Source: CAD feature listing. Evaluate the final solid. Frame: model axes, mm. A direction names the side the tool comes from. Coordinates: 2 decimals unless noted, no trailing zeros. Write each loop counter-clockwise with the first axis right and the second up, starting at its lowest first coordinate (ties: lowest second). Pieces come first, ordered by that corner, then holes. Notation, with made-up numbers: (71.5, -29.75) - (114.5, -29.75) arc R19 ccw to (114.5, -1.75) - close; hole circle Ø11 at (64, 53). An arc over 180 degrees is marked (long way). One line per item, written item: value.
from build123d import *

# Parameters (mm, degrees)
F0_W      = 42
F0_H      = 42
F1_DEPTH  = 39
F2_R      = 16
F3_DEPTH  = 22.1
F4_R      = 10
F5_DEPTH  = 3
F6_R      = 3
F7_DEPTH  = 16.3
F8_SIZE   = 5
F10_DEPTH = 12
F12_DEPTH = 3
F14_D     = 2.5
F14_DEPTH = 7
F14_TIP   = 0.7510757738


with BuildPart() as f1:
    # F0 (on Front) → F1 (new body)
    with BuildSketch(Plane.XZ):
        Rectangle(F0_W, F0_H)
    extrude(amount=F1_DEPTH)

    # F2 (on face) → F3 (join)
    with BuildSketch(Plane.XZ.offset(39)):
        Circle(F2_R)
    extrude(amount=F3_DEPTH)

    # F4 (on face) → F5 (join)
    with BuildSketch(Plane.XZ.offset(61.1)):
        Circle(F4_R)
    extrude(amount=F5_DEPTH)

    # F6 (on face) → F7 (join)
    with BuildSketch(Plane.XZ.offset(64.1)):
        Circle(F6_R)
    extrude(amount=F7_DEPTH)

    # F8
    f8_edges = [f1.edges().sort_by_distance(p)[0] for p in [
        (-21, -19.5, 21),
        (21, -19.5, 21),
        (21, -19.5, -21),
        (-21, -19.5, -21),
    ]]
    chamfer(f8_edges, length=F8_SIZE)

    # F9 (on face) → F10 (cut)
    with BuildSketch(Plane.XZ.offset(80.4)):
        with BuildLine():
            Line((-1.6583123952, 2.5), (1.6583123952, 2.5))
            ThreePointArc((1.6583123952, 2.5), (0, 3), (-1.6583123952, 2.5))
        make_face()
    extrude(amount=-F10_DEPTH, mode=Mode.SUBTRACT)

    # F11 (on face) → F12 (cut, through all)
    with BuildSketch(Plane.XZ.offset(64.1)):
        with BuildLine():
            Line((3.2817540292, 9.4461680322), (9.4461680322, 3.2817540292))
            ThreePointArc((9.4461680322, 3.2817540292), (7.0710678119, 7.0710678119), (3.2817540292, 9.4461680322))
        make_face()
        with BuildLine():
            ThreePointArc((-9.4461680322, -3.2817540292), (-7.0710678119, -7.0710678119), (-3.2817540292, -9.4461680322))
            Line((-3.2817540292, -9.4461680322), (-9.4461680322, -3.2817540292))
        make_face()
    extrude(amount=-F12_DEPTH, mode=Mode.SUBTRACT)

    # F14
    with Locations(Plane.XZ.offset(61.1)):
        with Locations((0, 13), (-13, 0), (0, -13), (13, 0)):
            Hole(F14_D / 2, depth=F14_DEPTH)
            with Locations((0, 0, -(F14_DEPTH + F14_TIP / 2))):  # 118° drill point
                Cone(0, F14_D / 2, F14_TIP, mode=Mode.SUBTRACT)


solid = f1.part
1) Section query A-A on y = -63. Output: boundary loops of the cut face in (x, z), then the cut area to 3 significant figures.
Values found:
outline: (-9.45, -3.28) - (-3.28, -9.45) arc R10 ccw to (9.45, 3.28) - (3.28, 9.45) arc R10 ccw to start
area: 302 mm2
2) Material intervals for line 1 (Z direction, x = 0, y = -59); line 2 (Y direction, x = -1.5, z = -11); line 3 (Y direction, x = -7, z = 4.5), sorted ascending.
Values found:
line 1: -16 to -14.25, -11.75 to 11.75, 14.25 to 16
line 2: -61.1 to 0
line 3: -64.1 to 0
3) Contact query for flat-ended pins moving along their axis: P1, Ø12, axis at y = -56.5, z = 12, coming from the -X side; P2, Ø10, axis at x = 0.5, y = -47, coming from the +Z side; P3, Ø1, axis at x = 9, z = -1, coming from the -Y side. Output: stop coordinate, or through.
Values found:
P1: x = -14.83
P2: z = 16
P3: y = -64.1
4) Section query B-B on x = 8. Output: boundary loops of the cut face in (y, z), then the cut area to 3 significant figures.
Values found:
outline: (-64.1, -6) - (-61.1, -6) - (-61.1, -13.86) - (-39, -13.86) - (-39, -21) - (0, -21) - (0, 21) - (-39, 21) - (-39, 13.86) - (-61.1, 13.86) - (-61.1, 4.73) - (-64.1, 4.73) - close
area: 2,280 mm2
5) Draft query along X for faces 4 (the flat face through (-6.32, -62.62, -6.41)), 5 (the flat face through (19, -19, 18)), 6 (the conical face through (-0.028, -53.479, -12.785)). Return one class per face: released by +X, released by -X, zero draft, split by the parting line, or undercut.
Values found:
face 4: released by -X
face 5: released by +X
face 6: undercut
6) Reachability of faces 1 (the flat face through (6.32, -62.62, 6.41)), 2 (the flat face through (19, -19, -18)), 3 (the flat face through (-2.4, -64.1, -2.1)) from +Z, -Z, +X, -X, +Y, -Y: full face, straight path, thin tool, end or side. Return the list, or none.
Values found:
face 1: +Z, +X, -Y
face 2: -Z, +X, +Y, -Y
face 3: -Y
7) Section query C-C on x = 18. Output: boundary loops of the cut face in (y, z).
Values found:
outline: (-39, -19) - (0, -19) - (0, 19) - (-39, 19) - close
